from build123d import *

# Parameters (mm, degrees)
SKETCH1_W           = 40
SKETCH1_H           = 40
BOSS_EXTRUDE1_DEPTH = 7
SKETCH3_R           = 2
CUT_EXTRUDE2_DEPTH  = 8
FILLET1_R           = 5
CUT_EXTRUDE7_DEPTH  = 5
SKETCH4_R           = 4
BOSS_EXTRUDE2_DEPTH = 36
SKETCH5_R           = 2
CUT_EXTRUDE8_DEPTH  = 5


with BuildPart() as part:
    # Sketch1 → Boss-Extrude1 (new body)
    with BuildSketch(Plane(origin=(0, 0, 0), x_dir=(1, 0, 0), z_dir=(0, 1, 0))):
        Rectangle(SKETCH1_W, SKETCH1_H)
    extrude(amount=BOSS_EXTRUDE1_DEPTH)

    # Sketch3 → Cut-Extrude2 (cut, through all)
    with BuildSketch(Plane(origin=(0, 7, 0), x_dir=(1, 0, 0), z_dir=(0, 1, 0))):
        with Locations((-10, 10)):
            Circle(SKETCH3_R)
        with Locations((10, 10)):
            Circle(SKETCH3_R)
        with Locations((-10, -10)):
            Circle(SKETCH3_R)
        with Locations((10, -10)):
            Circle(SKETCH3_R)
    extrude(amount=-CUT_EXTRUDE2_DEPTH, mode=Mode.SUBTRACT)

    # Fillet1
    fillet1_edges = [part.edges().sort_by_distance(p)[0] for p in [
        (20, 3.5, 20),
        (-20, 3.5, 20),
        (-20, 3.5, -20),
        (20, 3.5, -20),
    ]]
    fillet(fillet1_edges, radius=FILLET1_R)

    # Sketch2 → Cut-Extrude7 (cut)
    with BuildSketch(Plane(origin=(0, 0, 0), x_dir=(1, 0, 0), z_dir=(0, 1, 0))):
        Polygon((-5.843078062, -10), (-10, -10), (-10, -6.4), (-12.078460969, -6.4), (-14.156921938, -10), (-12.078460969, -13.6), (-7.921539031, -13.6), align=None)
        Polygon((10, -10), (5.843078062, -10), (7.921539031, -13.6), (12.078460969, -13.6), (14.156921938, -10), (12.078460969, -6.4), (10, -6.4), align=None)
        Polygon((7.921539031, -6.4), (5.843078062, -10), (10, -10), (10, -6.4), align=None)
        Polygon((-10, -6.4), (-10, -10), (-5.843078062, -10), (-7.921539031, -6.4), align=None)
        Polygon((-12.078460969, 6.4), (-10, 6.4), (-10, 10), (-5.843078062, 10), (-7.921539031, 13.6), (-12.078460969, 13.6), (-14.156921938, 10), align=None)
        Polygon((-10, 10), (-10, 6.4), (-7.921539031, 6.4), (-5.843078062, 10), align=None)
        Polygon((7.921539031, 6.4), (10, 6.4), (10, 10), (5.843078062, 10), align=None)
        Polygon((10, 10), (10, 6.4), (12.078460969, 6.4), (14.156921938, 10), (12.078460969, 13.6), (7.921539031, 13.6), (5.843078062, 10), align=None)
    extrude(amount=CUT_EXTRUDE7_DEPTH, mode=Mode.SUBTRACT)

    # Sketch4 → Boss-Extrude2 (add)
    with BuildSketch(Plane(origin=(0, 0, 0), x_dir=(1, 0, 0), z_dir=(0, 1, 0))):
        with Locations((0, -10.76)):
            Circle(SKETCH4_R)
    extrude(amount=-BOSS_EXTRUDE2_DEPTH)

    # Sketch5 → Cut-Extrude8 (cut)
    with BuildSketch(Plane(origin=(0, -36, 0), x_dir=(-1, 0, 0), z_dir=(0, -1, 0))):
        with Locations((0, -10.76)):
            Circle(SKETCH5_R)
    extrude(amount=-CUT_EXTRUDE8_DEPTH, mode=Mode.SUBTRACT)


solid = part.part
CAD build for the part. Positions are in the model's coordinates, mm. A direction names the side the tool comes from. Give positions to 0.01 mm unless a question says otherwise; leave off trailing zeros. Order: outer loops, then holes, each group sorted by start corner. A loop starts at its lowest first (then second) coordinate and runs counter-clockwise, first axis right, second up. Notation, with made-up numbers: (35.5, 38) -> (94.5, 38) arc R21 cw to (94.5, 68) -> close; hole circle Ø3 at (76.25, -15.75). An arc over 180 degrees is marked (long way). Return JSON: item names as keys, results as strings.
Q1. Flat gauge pins, fed straight in: pin 1 (1.5 mm diameter, centred on x = 4, z = -13.5, fed in from -Y); pin 2 (3 mm diameter, centred on x = 10, z = -10, fed in from +Y); pin 3 (3.5 mm diameter, centred on x = -10.5, z = -9.5, fed in from -Y); pin 4 (5 mm diameter, centred on y = -22.5, z = 14.5, fed in from -X). Where does each tip first touch, or does it go through?
Working result:
{"pin 1": "y = 0", "pin 2": "through", "pin 3": "y = 5", "pin 4": "x = -3.8"}
Q2. Mould opens along Z. For faces 1 (the face through (18, 4, -19)), 2 (the face through (-7, 2, 12)), 3 (the face through (10, 6, -12)), 4 (the face through (-19, 4, 18)) say: pulls with the +Z half, pulls with the -Z half, needs draft (parallel to the pull), parting line crosses it, or undercut.
Working result:
{"face 1": "pulls with the -Z half", "face 2": "undercut", "face 3": "undercut", "face 4": "pulls with the +Z half"}
Q3. Saw through at D-D (z = 10.76). Write the cut outline in (x, y), then the cut area to 3 significant figures.
Working result:
{"outline": "(-20, 0) -> (-13.72, 0) -> (-13.72, 5) -> (-11.85, 5) -> (-11.85, 7) -> (-20, 7) -> close; (-8.15, 5) -> (-6.28, 5) -> (-6.28, 0) -> (-4, 0) -> (-4, -36) -> (-2, -36) -> (-2, -31) -> (2, -31) -> (2, -36) -> (4, -36) -> (4, 0) -> (6.28, 0) -> (6.28, 5) -> (8.15, 5) -> (8.15, 7) -> (-8.15, 7) -> close; (11.85, 5) -> (13.72, 5) -> (13.72, 0) -> (20, 0) -> (20, 7) -> (11.85, 7) -> close", "area": "459 mm²"}
Q4. Drill centre lines: line 1 (Z direction, x = 12, y = 2); line 2 (X direction, y = 5.9, z = 10). Where is each one in solid material? Low to high.
Working result:
{"line 1": "-20 to -13.6, -6.4 to 6.4, 13.6 to 20", "line 2": "-20 to -12, -8 to 8, 12 to 20"}
Q5. Saw through at A-A (y = 2). Count the separate pieces of the cut face and the enclosed holes in it, then the cut area to 3 significant figures.
Working result:
{"separate pieces": "1", "enclosed holes": "4", "area": "1,400 mm²"}
Q6. Which spindle directions (+Z, -Z, +X, -X, +Y, -Y) get a long thin tool onto all of the face, cutting with end or side? Do faces 5 (the face through (0, 7, 0)), 6 (the face through (-10, 2, -13.6)). Say none if no direction does.
Working result:
{"face 5": "+Z, -Z, +X, -X, +Y", "face 6": "-Y"}
Q7. Saw through at B-B (x = 10). Write the cut outline in (y, z).
Working result:
{"outline": "(0, -20) -> (7, -20) -> (7, -12) -> (5, -12) -> (5, -13.6) -> (0, -13.6) -> close; (0, -6.4) -> (5, -6.4) -> (5, -8) -> (7, -8) -> (7, 8) -> (5, 8) -> (5, 6.4) -> (0, 6.4) -> close; (0, 13.6) -> (5, 13.6) -> (5, 12) -> (7, 12) -> (7, 20) -> (0, 20) -> close"}
Q8. Saw through at C-C (x = 0). Write the cut outline in (y, z), then the cut area to 3 significant figures.
Working result:
{"outline": "(-36, 6.76) -> (0, 6.76) -> (0, -20) -> (7, -20) -> (7, 20) -> (0, 20) -> (0, 14.76) -> (-36, 14.76) -> (-36, 12.76) -> (-31, 12.76) -> (-31, 8.76) -> (-36, 8.76) -> close", "area": "548 mm²"}
